Build history of the part. All positions in model axes, mm. A direction names the side the tool comes from. Round coordinates to 2 decimals unless told otherwise and drop trailing zeros. Write each loop counter-clockwise with the first axis right and the second up, starting at its lowest first coordinate (ties: lowest second). Pieces come first, ordered by that corner, then holes.
Item 1: Band-saw the part on A-A, the plane z = 3.6. Count the separate pieces of the cut face and the enclosed holes in it, then the cut area to 3 significant figures.
Item 2: Band-saw the part on C-C, the plane x = -32. Write the cut outline in (y, z), then the cut area to 3 significant figures.
Item 3: Band-saw the part on B-B, the plane y = 46.1. Write the cut outline in (x, z).
Item 4: Wall check: probe 1 along Y at (x, z) = (-15.5, 3.2); probe 2 along Y at (x, z) = (11, 4.15); probe 3 along Y at (x, z) = (-38, 2.1). Give the ranges that are in metal, low to high.
Item 5: 3-axis set-ups, long thin cutter, end or side, ignore diameter. For faces 4 (the flat face through (33.25, 37, 3)), 5 (the flat face through (-30, 43.6, 2)), 6 (the flat face through (1, -6, 5)): which of +Z, -Z, +X, -X, +Y, -Y reach the whole face in a straight line?
Item 6: Band-saw the part on D-D, the plane x = 15.5. Write the cut outline in (y, z), then the cut area to 3 significant figures.
Item 7: Drop flat-ended pins along their axis: pin 1 Ø1.5 at (x, z) = (-30, 1.5) entering from +Y; pin 2 Ø1.2 at (y, z) = (45.5, 3.5) entering from -X; pin 3 Ø1.5 at (y, z) = (38.5, 3) entering from +X. Give the stop position or say it passes through.
Item 8: Mould opens along X. For faces 1 (the cylindrical face through (-46.39, -40.18, 2.54)), 2 (the cylindrical face through (46.58, -39.99, 2.54)), 3 (the cylindrical face through (14.026, 16.452, 2.535)) say: +X half, -X half, draft (parallel to the pull), parting line (faces both ways), or undercut.
```python
from build123d import *

# Parameters (mm, degrees)
Y_KSEKLIK_EKSTR_ZYON1_DEPTH = 5
IZIM2_R                     = 2.5
IZIM2_R_2                   = 2
KES_EKSTR_ZYON1_DEPTH       = 10
IZIM4_W                     = 66.5
IZIM4_H                     = 7
KES_EKSTR_ZYON3_DEPTH       = 5
RADYUS1_R                   = 12


with BuildPart() as part:
    # Çizim1 → Yükseklik-Ekstrüzyon1 (new body)
    with BuildSketch(Plane.XY):
        Polygon((21, 43.6), (50, 43.6), (50, -43.6), (-50, -43.6), (-50, 43.6), (-21, 43.6), (-21, 47.6), (-17, 51.6), (17, 51.6), (21, 47.6), align=None)
    extrude(amount=Y_KSEKLIK_EKSTR_ZYON1_DEPTH)

    # Çizim2 → Kes-Ekstrüzyon1 (cut)
    with BuildSketch(Plane.XY.offset(5)):
        with Locations((38, -31.6)):
            Circle(IZIM2_R)
        with Locations((38, 31.6)):
            Circle(IZIM2_R)
        with Locations((-15.5, 46.1)):
            Circle(IZIM2_R_2)
        with Locations((15.5, 46.1)):
            Circle(IZIM2_R_2)
        with Locations((15.5, 15.1)):
            Circle(IZIM2_R_2)
        with Locations((-15.5, 15.1)):
            Circle(IZIM2_R_2)
        with Locations((-38, 31.6)):
            Circle(IZIM2_R)
        with Locations((-38, -31.6)):
            Circle(IZIM2_R)
    extrude(amount=-KES_EKSTR_ZYON1_DEPTH, mode=Mode.SUBTRACT)

    # Çizim4 → Kes-Ekstrüzyon3 (cut)
    with BuildSketch(Plane.XY.offset(5)):
        with Locations((0, 37.1)):
            Rectangle(IZIM4_W, IZIM4_H)
    extrude(amount=-KES_EKSTR_ZYON3_DEPTH, mode=Mode.SUBTRACT)

    # Radyus1
    radyus1_edges = [part.edges().sort_by_distance(p)[0] for p in [
        (50, -43.6, 2.5),
        (-50, -43.6, 2.5),
        (-50, 43.6, 2.5),
        (50, 43.6, 2.5),
    ]]
    fillet(radyus1_edges, radius=RADYUS1_R)


solid = part.part
```
Results:
1. separate pieces: 1
1. enclosed holes: 9
1. area: 8,320 mm2
2. outline: (-43.6, 0) - (33.6, 0) - (33.6, 5) - (-43.6, 5) - close; (40.6, 0) - (43.6, 0) - (43.6, 5) - (40.6, 5) - close
2. area: 401 mm2
3. outline: (-21, 0) - (-17.5, 0) - (-17.5, 5) - (-21, 5) - close; (-13.5, 0) - (13.5, 0) - (13.5, 5) - (-13.5, 5) - close; (17.5, 0) - (21, 0) - (21, 5) - (17.5, 5) - close
4. probe 1: y = -43.6 to 13.1, 17.1 to 33.6, 40.6 to 44.1, 48.1 to 51.6
4. probe 2: y = -43.6 to 33.6, 40.6 to 51.6
4. probe 3: y = -43.6 to -34.1, -29.1 to 29.1, 34.1 to 43.6
5. face 4: +Z, -Z
5. face 5: +Z, -Z, -X, +Y
5. face 6: +Z, +X, -X, +Y, -Y
6. outline: (-43.6, 0) - (13.1, 0) - (13.1, 5) - (-43.6, 5) - close; (17.1, 0) - (33.6, 0) - (33.6, 5) - (17.1, 5) - close; (40.6, 0) - (44.1, 0) - (44.1, 5) - (40.6, 5) - close; (48.1, 0) - (51.6, 0) - (51.6, 5) - (48.1, 5) - close
6. area: 401 mm2
7. pin 1: stops at y = 43.6
7. pin 2: stops at x = -21
7. pin 3: stops at x = 48.3
8. face 1: -X half
8. face 2: +X half
8. face 3: undercut
